from build123d import *

# Parameters (mm, degrees)
F1_DEPTH = 20
F2_R     = 2


# Not quite as in the source:
# - a feature names something its author has since deleted; it is built from what else it names


with BuildPart() as f1:
    # F0 (on Top) → F1 (new body)
    with BuildSketch(Plane.XY):
        with BuildLine():
            ThreePointArc((-33.4013422072, 19.5177844279), (-33.1069150162, 19.1649980234), (-33.0013422072, 18.7177844279))
            Line((-33.0013422072, 18.7177844279), (-33.0013422072, 17.7177844279))
            ThreePointArc((-33.0013422072, 17.7177844279), (-32.4155557696, 16.3035708655), (-31.0013422072, 15.7177844279))
            Line((-31.0013422072, 15.7177844279), (-23.5013422072, 15.7177844279))
            ThreePointArc((-23.5013422072, 15.7177844279), (-22.794235426, 15.424891209), (-22.5013422072, 14.7177844279))
            Line((-22.5013422072, 14.7177844279), (-22.5013422072, 13.4677844279))
            ThreePointArc((-22.5013422072, 13.4677844279), (-22.794235426, 12.7606776467), (-23.5013422072, 12.4677844279))
            Line((-23.5013422072, 12.4677844279), (-32.781970528, 12.4677844279))
            ThreePointArc((-32.781970528, 12.4677844279), (-33.4890773091, 12.174891209), (-33.781970528, 11.4677844279))
            ThreePointArc((-33.781970528, 11.4677844279), (-34.0748637468, 10.7606776467), (-34.781970528, 10.4677844279))
            Line((-34.781970528, 10.4677844279), (-35.5013422072, 10.4677844279))
            ThreePointArc((-35.5013422072, 10.4677844279), (-36.2084489884, 10.174891209), (-36.5013422072, 9.4677844279))
            Line((-36.5013422072, 9.4677844279), (-36.5013422072, 2.9677844279))
            Line((-36.5013422072, 2.9677844279), (-36.5013422072, 1.0177844279))
            Line((-36.5013422072, 1.0177844279), (-38.5013422072, 1.0177844279))
            Line((-38.5013422072, 1.0177844279), (-46.5013422072, 1.0177844279))
            Line((-46.5013422072, 1.0177844279), (-46.5013422072, 0.5177844279))
            Line((-46.5013422072, 0.5177844279), (-46.5013422072, -1.4822155721))
            ThreePointArc((-46.5013422072, -1.4822155721), (-45.9155557696, -2.8964291345), (-44.5013422072, -3.4822155721))
            Line((-44.5013422072, -3.4822155721), (-32.935840724, -3.4822155721))
            ThreePointArc((-32.935840724, -3.4822155721), (-30.679965917, -3.0419843493), (-28.7551266184, -1.7858918573))
            Line((-28.7551266184, -1.7858918573), (-18.3206281016, 8.3504781304))
            ThreePointArc((-18.3206281016, 8.3504781304), (-16.9748476295, 10.3179485849), (-16.5013422072, 12.6541544156))
            Line((-16.5013422072, 12.6541544156), (-16.5013422072, 16.7177844279))
            ThreePointArc((-16.5013422072, 16.7177844279), (-18.2587015201, 20.960425115), (-22.5013422072, 22.7177844279))
            Line((-22.5013422072, 22.7177844279), (-36.0013422072, 22.7177844279))
            ThreePointArc((-36.0013422072, 22.7177844279), (-38.1226625508, 21.8391047714), (-39.0013422072, 19.7177844279))
            Line((-39.0013422072, 19.7177844279), (-39.0013422072, 19.2177844279))
            Line((-39.0013422072, 19.2177844279), (-38.8548955978, 19.3642310373))
            ThreePointArc((-38.8548955978, 19.3642310373), (-38.5013422072, 19.5106776467), (-38.1477888166, 19.3642310373))
            Line((-38.1477888166, 19.3642310373), (-38.0013422072, 19.2177844279))
            Line((-38.0013422072, 19.2177844279), (-37.8548955978, 19.3642310373))
            ThreePointArc((-37.8548955978, 19.3642310373), (-37.5013422072, 19.5106776467), (-37.1477888166, 19.3642310373))
            Line((-37.1477888166, 19.3642310373), (-37.0013422072, 19.2177844279))
            Line((-37.0013422072, 19.2177844279), (-36.8463774903, 19.3727491447))
            ThreePointArc((-36.8463774903, 19.3727491447), (-36.498920301, 19.5191585891), (-36.1479965135, 19.3812647196))
            Line((-36.1479965135, 19.3812647196), (-35.9763422072, 19.2177844279))
            Line((-35.9763422072, 19.2177844279), (-35.8449793172, 19.3557154623))
            ThreePointArc((-35.8449793172, 19.3557154623), (-35.4951018479, 19.5107392214), (-35.1380827655, 19.3729568416))
            Line((-35.1380827655, 19.3729568416), (-35.0041172482, 19.2453706347))
            ThreePointArc((-35.0041172482, 19.2453706347), (-34.9722907986, 19.2249367588), (-34.935151731, 19.2177844279))
            Line((-34.935151731, 19.2177844279), (-34.5013422072, 19.2177844279))
            ThreePointArc((-34.5013422072, 19.2177844279), (-34.2777354094, 19.2705708324), (-34.1013422072, 19.4177844279))
            ThreePointArc((-34.1013422072, 19.4177844279), (-33.7720528853, 19.6127591747), (-33.4013422072, 19.5177844279))
        make_face()
    extrude(amount=F1_DEPTH)

    # F2
    f2_edges = [f1.edges().sort_by_distance(p)[0] for p in [
        (-29.251342, 22.717784, 20),
        (-29.251342, 22.717784, 0),
    ]]
    fillet(f2_edges, radius=F2_R)


solid = f1.part
Read the model definition and answer for the solid it produces. Units are mm, in the model's axes. A direction names the side the tool comes from. Coordinates: 2 decimals unless noted, no trailing zeros. Answer as a JSON object with one key per item and string values.
1) The mould has two halves that part along Y. Classify faces 1 (the face through (-29.346, 22.147, 0.601)), 2 (the face through (-32.43, 16.32, 9.86)), 3 (the face through (-30.71, -3.054, 9.888)): released by +Y, released by -Y, zero draft, split by the parting line, or undercut.
Model answer:
{"face 1": "released by +Y", "face 2": "undercut", "face 3": "released by -Y"}
2) Consider line 1 along Y through (x, z) = (-23, 7.5); line 2 along X through (y, z) = (14.5, 2.5); line 3 along Y through (x, z) = (-26.5, 12.5). Determine where each line is inside the solid, lowest interval first. Write a range as from..to.
Model answer:
{"line 1": "y = 3.8..12.6, 15.58..22.72", "line 2": "x = -22.5..-16.5", "line 3": "y = 0.4..12.47, 15.72..22.72"}
3) A tool of negligible diameter and unlimited length cuts with its end or side. For faces 4 (the face through (-36.501, 5, 10)), 5 (the face through (-45.93, -0.25, 19.4)), from which of +Z, -Z, +X, -X, +Y, -Y can it reach the whole face along a straight path? Write none if from no direction.
Model answer:
{"face 4": "+Z, -Z, -X", "face 5": "+Z, -X, +Y, -Y"}
4) Each of these flat-tipped pins is pushed along its axis until it touches: pin 1 (1 mm diameter, centred on y = 18, z = 5.5, fed in from +X); pin 2 (1.1 mm diameter, centred on y = 18, z = 13, fed in from -X); pin 3 (4 mm diameter, centred on y = 3, z = 8.5, fed in from +X); pin 4 (8 mm diameter, centred on x = -34, y = 7, fed in from -Z). Where does it stop, or does it pass through?
Model answer:
{"pin 1": "stops at x = -16.55", "pin 2": "stops at x = -33", "pin 3": "stops at x = -21.77", "pin 4": "stops at z = 0"}
